```python
from build123d import *

# Parameters (mm, degrees)
SKETCH_1_R                = 2
F_12MM_5_M4_DEPTH         = 5
EXTRUDE_START             = 5
SKETCH_2_R                = 5.75
SKETCH_2_R_2              = 3
EXTRUDE_11_5_6_13_DEPTH   = 13
CUT_EXTRUDE_M4_DEPTH      = 21.199009877
CUT_EXTRUDE_M4_DEPTH_BACK = 21.199009877
SKETCH_3_R                = 1.65


with BuildPart() as part:
    # 草图1 → 轮毂端六角12mm_厚5_中心M4孔简化 (new body)
    with BuildSketch(Plane.XY):
        Polygon((6.92820323, 0), (3.464101615, 6), (-3.464101615, 6), (-6.92820323, 0), (-3.464101615, -6), (3.464101615, -6), align=None)
        Circle(SKETCH_1_R, mode=Mode.SUBTRACT)
    extrude(amount=F_12MM_5_M4_DEPTH)

    # 草图2 → 电机端_外径11.5_孔径6_长13 (add)
    with BuildSketch(Plane.XY.offset(EXTRUDE_START)):
        with Locations(Location((0, 0, 0), (0, 0, 180))):
            Circle(SKETCH_2_R)
        with Locations(Location((0, 0, 0), (0, 0, 180))):
            Circle(SKETCH_2_R_2, mode=Mode.SUBTRACT)
    extrude(amount=EXTRUDE_11_5_6_13_DEPTH)

    # 草图3 → M4紧定螺钉底孔_牙型简化 (cut, two sides: drawn at the far end of the back side and taken through both)
    with BuildSketch(Plane(origin=(0, 0, 0), x_dir=(0, 0, -1), z_dir=(1, 0, 0)).offset(-CUT_EXTRUDE_M4_DEPTH_BACK)):
        with Locations(Location((-11.5, 0, 0), (0, 0, 180))):
            Circle(SKETCH_3_R)
    extrude(amount=CUT_EXTRUDE_M4_DEPTH + CUT_EXTRUDE_M4_DEPTH_BACK, mode=Mode.SUBTRACT)


solid = part.part
```
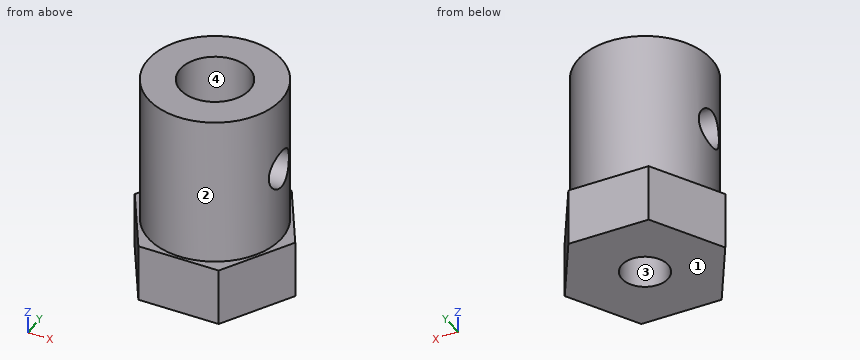
Model file for the job. Use its own axes, mm. Face numbers are marked on the shaded views. Give positions to 0.01 mm unless a question says otherwise; leave off trailing zeros. Loops run counter-clockwise (first coordinate to the right, second up) from the corner with the lowest first, then second, coordinate; pieces in that order, holes last. Notation, with made-up numbers: (30, 24.5) - (73, 24.5) arc R6 ccw to (73, 30.5) - close; hole circle Ø9 at (-38, -14.75). An arc over 180 degrees is marked (long way). One line per item, written item: value. Start each with the question number.
1. Pull direction X, two halves, no side cores. Call the marked faces 1, 2, 3 and 4: pulls with the +X half, pulls with the -X half, needs draft (parallel to the pull), parting line crosses it, or undercut.
2. Slice it at B-B (z = 11.5). List the corners of the cut face in (x, y).
3. Slice it at D-D (x = -4). List the corners of the cut face in (y, z).
4. Probe L1, parallel to X at y = 1.75, z = 10.5; L2, parallel to X at y = -0.25, z = 16.5; L3, parallel to Y at x = -2.5, z = 13.75. List the from-to ranges inside material, lowest first. Write a range as from..to.
5. Slice it at C-C (y = -0.75). List the corners of the cut face in (x, z), plus the area to 3 significant figures.
6. Pin check, flat tips, straight feed: pin 1 (4 mm diameter, centred on y = 0, z = 11.5, fed in from -X); pin 2 (2 mm diameter, centred on x = -4.5, z = 12, fed in from +Y); pin 3 (2 mm diameter, centred on y = -1.5, z = 9, fed in from -X). Stop position of each tip, or through.
7. Slice it at A-A (x = 0). List the corners of the cut face in (y, z).
Solution:
1. face 1: needs draft
1. face 2: parting line crosses it
1. face 3: undercut
1. face 4: undercut
2. outline: (-5.51, -1.65) arc R5.75 ccw to (5.51, -1.65) - (2.51, -1.65) arc R3 cw to (-2.51, -1.65) - close; (-5.51, 1.65) - (-2.51, 1.65) arc R3 cw to (2.51, 1.65) - (5.51, 1.65) arc R5.75 ccw to start
3. outline: (-5.07, 0) - (5.07, 0) - (5.07, 5) - (4.13, 5) - (4.13, 18) - (-4.13, 18) - (-4.13, 5) - (-5.07, 5) - close; hole circle Ø3.3 at (0, 11.5)
4. L1: x = -5.48..-2.44, 2.44..5.48
4. L2: x = -5.74..-2.99, 2.99..5.74
4. L3: y = -5.18..-1.66, 1.66..5.18
5. outline: (-6.5, 0) - (-1.85, 0) - (-1.85, 5) - (-2.9, 5) - (-2.9, 10.03) - (-5.7, 10.03) - (-5.7, 5) - (-6.5, 5) - close; (-5.7, 12.97) - (-2.9, 12.97) - (-2.9, 18) - (-5.7, 18) - close; (1.85, 0) - (6.5, 0) - (6.5, 5) - (5.7, 5) - (5.7, 10.03) - (2.9, 10.03) - (2.9, 5) - (1.85, 5) - close; (2.9, 12.97) - (5.7, 12.97) - (5.7, 18) - (2.9, 18) - close
5. area: 103 mm^2
6. pin 1: stops at x = -5.75
6. pin 2: stops at y = 4.56
6. pin 3: stops at x = -5.73
7. outline: (-6, 0) - (-2, 0) - (-2, 5) - (-3, 5) - (-3, 18) - (-5.75, 18) - (-5.75, 5) - (-6, 5) - close; (2, 0) - (6, 0) - (6, 5) - (5.75, 5) - (5.75, 18) - (3, 18) - (3, 5) - (2, 5) - close
